Geometry: final body of the model. Coordinates: model frame, mm. A direction names the side the tool comes from. Give positions to 0.01 mm unless a question says otherwise; leave off trailing zeros. Loops run counter-clockwise (first coordinate to the right, second up) from the corner with the lowest first, then second, coordinate; pieces in that order, holes last. Notation, with made-up numbers: M 2,-23.5 L 40,-23.5 A12 ccw 40,-4.5 Z; hole C 34.5,11.5 d3. An arc over 180 degrees is marked long. One line per question, with ' | ' between items. Start each with the question number.
from build123d import *

# Parameters (mm, degrees)
SKETCH_1_R          = 2
EXTRUDE_1_DEPTH     = 2
SKETCH_6_W          = 22
SKETCH_6_H          = 10
EXTRUDE_5_DEPTH     = 2
CHAMFER_2_SIZE      = 2
CHAMFER_3_SIZE      = 4
SKETCH_7_R          = 3
CUT_EXTRUDE_2_DEPTH = 35.770677301


with BuildPart() as part:
    # Sketch 1 → Extrude 1 (new body)
    with BuildSketch(Plane.XY):
        with BuildLine():
            Line((0, 0), (18, 0))
            ThreePointArc((18, 0), (23, 5), (18, 10))
            Line((18, 10), (0, 10))
            Line((0, 10), (0, 0))
        make_face()
        with Locations((18, 5)):
            Circle(SKETCH_1_R, mode=Mode.SUBTRACT)
    extrude(amount=EXTRUDE_1_DEPTH)


with BuildPart() as body_2:
    # Mirror 1: mirrored copy
    add(part.part.mirror(Plane.XY.offset(11)))


with BuildPart() as part_1:
    add(part.part)

    add(body_2.part)  # Extrude 5 merges body 2
    # Sketch 6 → Extrude 5 (add)
    with BuildSketch(Plane.ZY):
        with Locations((11, 5)):
            Rectangle(SKETCH_6_W, SKETCH_6_H)
    extrude(amount=EXTRUDE_5_DEPTH)

    # Chamfer 2
    chamfer_2_edges = [part_1.edges().sort_by_distance(p)[0] for p in [
        (-2, 5, 0),
        (-2, 5, 22),
    ]]
    chamfer(chamfer_2_edges, length=CHAMFER_2_SIZE)

    # Chamfer 3
    chamfer_3_edges = [part_1.edges().sort_by_distance(p)[0] for p in [
        (0, 5, 20),
        (0, 5, 2),
    ]]
    chamfer(chamfer_3_edges, length=CHAMFER_3_SIZE)

    # Sketch 7 → Cut-Extrude 2 (cut, through all)
    with BuildSketch(Plane.ZY.offset(2)):
        with Locations((11, 5)):
            Circle(SKETCH_7_R)
    extrude(amount=-CUT_EXTRUDE_2_DEPTH, mode=Mode.SUBTRACT)


solid = part_1.part
Q1. Draft query along Z for faces 3 (the flat face through (2, 5, 18)), 4 (the cylindrical face through (-1, 3.2, 8.6)), 5 (the cylindrical face through (23, 5, 21)), 6 (the flat face through (12, 5, 0)). Return one class per face: released by +Z, released by -Z, zero draft, split by the parting line, or undercut.
Q2. Section D-D, the plane z = 15. Output: boundary loops of the cut face in (x, y).
Q3. Section B-B, the plane z = 11. Output: boundary loops of the cut face in (x, y).
Q4. Material intervals for L1, parallel to Z at x = 15.5, y = 1.5; L2, parallel to Y at x = 18, z = 1.35; L3, parallel to Y at x = -0.35, z = 11, sorted ascending.
Q5. Section C-C, the plane y = 5. Output: boundary loops of the cut face in (x, z).
Q6. Contact query for flat-ended pins moving along their axis: pin 1 (12 mm diameter, centred on x = 12.5, z = 4.5, fed in from -Y); pin 2 (5 mm diameter, centred on y = 4.5, z = 11.5, fed in from +X). Output: stop coordinate, or through.
Q7. Set-up query: faces 1 (the flat face through (13, 5, 20)), 2 (the flat face through (-1, 10, 9)). Return all of +Z, -Z, +X, -X, +Y, -Y with unobstructed straight access to the full face (end or side cutting, diameter ignored); none if empty.
Q8. Section A-A, the plane x = 11.25. Output: boundary loops of the cut face in (y, z), plus the area to 3 significant figures.
Model answer:
1) face 3: undercut | face 4: undercut | face 5: zero draft | face 6: released by -Z
2) outline: M -2,0 L 0,0 L 0,10 L -2,10 Z
3) outline: M -2,0 L 0,0 L 0,2 L -2,2 Z; M -2,8 L 0,8 L 0,10 L -2,10 Z
4) L1: z = 0 to 2, 20 to 22 | L2: y = 0 to 3, 7 to 10 | L3: y = 0 to 2, 8 to 10
5) outline: M -2,2 L 0,0 L 16,0 L 16,2 L 4,2 L 0,6 L 0,8 L -2,8 Z; M -2,14 L 0,14 L 0,16 L 4,20 L 16,20 L 16,22 L 0,22 L -2,20 Z; M 20,0 L 23,0 L 23,2 L 20,2 Z; M 20,20 L 23,20 L 23,22 L 20,22 Z
6) pin 1: stops at y = 0 | pin 2: stops at x = 0
7) face 1: +X, +Y, -Y | face 2: +Z, -Z, +X, -X, +Y
8) outline: M 0,0 L 10,0 L 10,2 L 0,2 Z; M 0,20 L 10,20 L 10,22 L 0,22 Z | area: 40.0 mm^2
